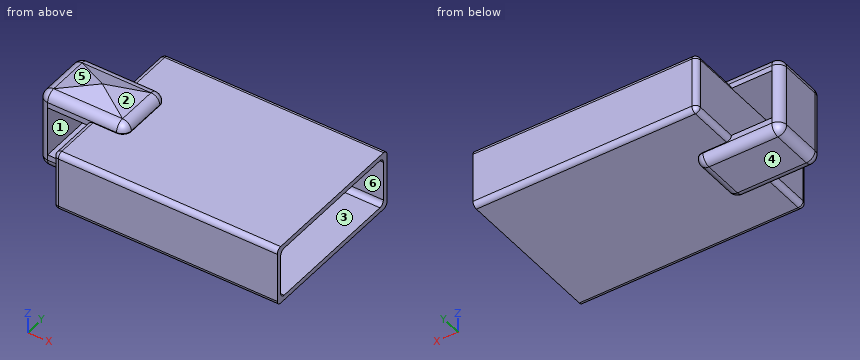
```python
from build123d import *

# Parameters (mm, degrees)
F0_W      = 17.2212
F0_H      = 12.2174
F2_DEPTH  = 2.2987
F1_W      = 6.6548
F1_H      = 4.5212
F3_DEPTH  = 3.0226
F4_R      = 0.67818
F5_R      = 0.381
F3_FACE_W = 5.29844
F3_FACE_H = 3.16484
F8_W      = 3.10642
F8_H      = 3.8354
F9_DEPTH  = 4.5212
F11_DEPTH = 16.8402
F12_R     = 0.381


with BuildPart() as f2:
    # F0 (on Top) → F2 (new body, symmetric)
    with BuildSketch(Plane.XY):
        Rectangle(F0_W, F0_H)
    extrude(amount=F2_DEPTH, both=True)

    # F1 (on Top) → F3 (join, symmetric)
    with BuildSketch(Plane.XY):
        with Locations((-9.0678, 0)):
            Rectangle(F1_W, F1_H)
    extrude(amount=F3_DEPTH, both=True)

    # F4
    f4_edges = [f2.edges().sort_by_distance(p)[0] for p in [
        (-9.0678, 2.2606, 3.0226),
        (-9.0678, 2.2606, -3.0226),
        (-9.0678, -2.2606, 3.0226),
        (-9.0678, -2.2606, -3.0226),
        (-5.7404, 0, -3.0226),
        (-5.7404, 0, 3.0226),
        (-12.3952, -2.2606, 0),
        (-12.3952, 2.2606, 0),
        (-12.3952, 0, -3.0226),
        (-12.3952, 0, 3.0226),
        (-5.7404, 2.2606, -2.66065),
        (-5.7404, 2.2606, 2.66065),
        (-5.7404, -2.2606, 2.66065),
        (-5.7404, -2.2606, -2.66065),
    ]]
    fillet(f4_edges, radius=F4_R)

    # F5
    f5_edges = [f2.edges().sort_by_distance(p)[0] for p in [
        (0, 6.1087, 2.2987),
        (0, 6.1087, -2.2987),
        (-8.6106, 6.1087, 0),
        (-8.6106, -4.18465, 2.2987),
        (-8.6106, 4.18465, 2.2987),
        (-8.6106, -4.18465, -2.2987),
        (-8.6106, 4.18465, -2.2987),
        (-8.6106, -6.1087, 0),
        (0, -6.1087, 2.2987),
        (0, -6.1087, -2.2987),
    ]]
    fillet(f5_edges, radius=F5_R)

    # F3_face (on face) → F7 section 0
    with BuildSketch(Plane(origin=(-9.0678, 0, 3.0226), x_dir=(1, 0, 0), z_dir=(0, 0, 1)), mode=Mode.PRIVATE) as f7_s0:
        Rectangle(F3_FACE_W, F3_FACE_H)
    loft([f7_s0.sketch, Vertex(-9.0678, 0, 3.5814)])

    # F8 (on face) → F9 (cut)
    with BuildSketch(Plane.XZ.offset(2.2606)):
        with Locations((-10.16381, 0)):
            Rectangle(F8_W, F8_H)
    extrude(amount=-F9_DEPTH, mode=Mode.SUBTRACT)

    # F10 (on face) → F11 (cut)
    with BuildSketch(Plane.YZ.offset(8.6106)):
        Polygon((5.7023, 1.9177), (0, 1.9177), (-5.7277, 1.9177), (-5.7277, 0), (-5.7277, -1.9177), (0, -1.9177), (5.7023, -1.9177), align=None)
    extrude(amount=-F11_DEPTH, mode=Mode.SUBTRACT)

    # F12
    f12_edges = [f2.edges().sort_by_distance(p)[0] for p in [
        (0.1905, 5.7023, 1.9177),
        (0.1905, -5.7277, 1.9177),
        (0.1905, -5.7277, -1.9177),
        (0.1905, 5.7023, -1.9177),
    ]]
    fillet(f12_edges, radius=F12_R)


solid = f2.part
```
Can you work these out from the model? Positions are in its coordinate system, mm. Face numbers are marked on the shaded views. A direction names the side the tool comes from. Round coordinates to 2 decimals unless told otherwise and drop trailing zeros. Loops run counter-clockwise (first coordinate to the right, second up) from the corner with the lowest first, then second, coordinate; pieces in that order, holes last. Notation, with made-up numbers: M 23.5,-37 L 49.5,-37 A22 cw 49.5,-7 Z; hole C -9,27 d4. An arc over 180 degrees is marked long. Answer as a JSON object with one key per item and string values. Group by question number.
Q1. Imagine slicing it at B-B, the plane y = 2.75. Please give me the cut outline in (x, z).
Q2. Imagine slicing it at C-C, the plane z = 0.75. Please give me the cut outline in (x, y).
Q3. Imagine slicing it at D-D, the plane x = 2.25. Please give me the cut outline in (y, z), then the cut area to 3 significant figures.
Q4. We'd pull the mould along Z, two halves only. Please class the marked faces 4, 5 and 6: +Z half, -Z half, draft (parallel to the pull), parting line (faces both ways), or undercut.
Q5. Please list where these lines run through material, in increasing order: L1, parallel to X at y = 0.5, z = -1.75; L2, parallel to Z at x = 1.5, y = -4.5; L3, parallel to Y at x = -5.75, z = -0.75.
Q6. Will these pins go through, and if not, where does the flat tip stop? pin 1 (2 mm diameter, centred on x = -3.5, y = 3, fed in from +Z); pin 2 (3 mm diameter, centred on x = -2.5, y = -0.5, fed in from -Z); pin 3 (3 mm diameter, centred on x = -10, y = -2.5, fed in from +Z).
Q7. On a 3-axis mill with a long thin cutter (end or side, diameter ignored), from which of +Z, -Z, +X, -X, +Y, -Y can I reach the whole of each face in a straight line? I mean the marked faces 1, 2 and 3. Say none if no direction works.
Q8. Imagine slicing it at A-A, the plane x = -10.75. Please give me the cut outline in (y, z), then the cut area to 3 significant figures.
Findings:
{
 "1": {"outline": "M -8.61,-1.92 A0.38 ccw -8.23,-2.3 L 8.61,-2.3 L 8.61,-1.92 L -8.23,-1.92 L -8.23,1.92 L 8.61,1.92 L 8.61,2.3 L -8.23,2.3 A0.38 ccw -8.61,1.92 Z"},
 "2": {"outline": "M -12.4,-1.58 A0.68 ccw -11.72,-2.26 L -11.72,2.26 A0.68 ccw -12.4,1.58 Z; M -8.61,-5.73 A0.38 ccw -8.23,-6.11 L 8.61,-6.11 L 8.61,-5.73 L -8.23,-5.73 L -8.23,5.7 L 8.61,5.7 L 8.61,6.11 L -8.23,6.11 A0.38 ccw -8.61,5.73 Z"},
 "3": {"outline": "M -6.11,-1.92 A0.38 ccw -5.73,-2.3 L 5.73,-2.3 A0.38 ccw 6.11,-1.92 L 6.11,1.92 A0.38 ccw 5.73,2.3 L -5.73,2.3 A0.38 ccw -6.11,1.92 Z; hole M -5.73,-1.54 A0.38 ccw -5.35,-1.92 L 5.32,-1.92 A0.38 ccw 5.7,-1.54 L 5.7,1.54 A0.38 ccw 5.32,1.92 L -5.35,1.92 A0.38 ccw -5.73,1.54 Z", "area": "12.3 mm2"},
 "4": {"face 4": "-Z half", "face 5": "+Z half", "face 6": "undercut"},
 "5": {"L1": "x = -12.4 to -11.72, -8.61 to -8.23", "L2": "z = -2.3 to -1.92, 1.92 to 2.3", "L3": "y = -6.11 to -5.73, 5.7 to 6.11"},
 "6": {"pin 1": "stops at z = 2.3", "pin 2": "stops at z = -2.3", "pin 3": "stops at z = 3.23"},
 "7": {"face 1": "+Y, -Y", "face 2": "+Z, +X, +Y, -Y", "face 3": "+X"},
 "8": {"outline": "M -2.26,-2.34 A0.68 ccw -1.58,-3.02 L 1.58,-3.02 A0.68 ccw 2.26,-2.34 L 2.26,-1.92 L -2.26,-1.92 Z; M -2.26,1.92 L 2.26,1.92 L 2.26,2.34 A0.68 ccw 1.58,3.02 L 1,3.23 L -1,3.23 L -1.58,3.02 A0.68 ccw -2.26,2.34 Z", "area": "10.1 mm2"}
}
